from build123d import *

# Parameters (mm, degrees)
SKETCH1_W           = 45
SKETCH1_H           = 45
BOSS_EXTRUDE1_DEPTH = 48
SKETCH2_W           = 7
SKETCH2_H           = 3
CUT_EXTRUDE1_DEPTH  = 15
SKETCH3_R           = 3
CUT_EXTRUDE2_DEPTH  = 8
SKETCH4_W           = 18.249611446
SKETCH4_H           = 11.178416291
CUT_EXTRUDE3_DEPTH  = 2
BOSS_EXTRUDE2_DEPTH = 5


with BuildPart() as part:
    # Sketch1 → Boss-Extrude1 (new body)
    with BuildSketch(Plane(origin=(0, 0, 0), x_dir=(1, 0, 0), z_dir=(0, 1, 0))):
        with Locations((22.5, 22.5)):
            Rectangle(SKETCH1_W, SKETCH1_H)
    extrude(amount=BOSS_EXTRUDE1_DEPTH)

    # Sketch2 → Cut-Extrude1 (cut)
    with BuildSketch(Plane(origin=(0, 48, 0), x_dir=(1, 0, 0), z_dir=(0, 1, 0))):
        with Locations((5.5, 1.5)):
            Rectangle(SKETCH2_W, SKETCH2_H)
        with Locations((14, 1.5)):
            Rectangle(SKETCH2_W, SKETCH2_H)
        with Locations((22.5, 1.5)):
            Rectangle(SKETCH2_W, SKETCH2_H)
        with Locations((31, 1.5)):
            Rectangle(SKETCH2_W, SKETCH2_H)
        with Locations((39.5, 1.5)):
            Rectangle(SKETCH2_W, SKETCH2_H)
        with Locations((39.5, 43.5)):
            Rectangle(SKETCH2_W, SKETCH2_H)
        with Locations((31, 43.5)):
            Rectangle(SKETCH2_W, SKETCH2_H)
        with Locations((22.5, 43.5)):
            Rectangle(SKETCH2_W, SKETCH2_H)
        with Locations((14, 43.5)):
            Rectangle(SKETCH2_W, SKETCH2_H)
        with Locations((5.5, 43.5)):
            Rectangle(SKETCH2_W, SKETCH2_H)
    extrude(amount=-CUT_EXTRUDE1_DEPTH, mode=Mode.SUBTRACT)

    # Sketch3 → Cut-Extrude2 (cut)
    with BuildSketch(Plane(origin=(0, 48, 0), x_dir=(1, 0, 0), z_dir=(0, 1, 0))):
        with Locations((5.5, 8)):
            Circle(SKETCH3_R)
        with Locations((14, 8)):
            Circle(SKETCH3_R)
        with Locations((22.5, 8)):
            Circle(SKETCH3_R)
        with Locations((31, 8)):
            Circle(SKETCH3_R)
        with Locations((39.5, 8)):
            Circle(SKETCH3_R)
        with Locations((39.5, 37)):
            Circle(SKETCH3_R)
        with Locations((31, 37)):
            Circle(SKETCH3_R)
        with Locations((22.5, 37)):
            Circle(SKETCH3_R)
        with Locations((14, 37)):
            Circle(SKETCH3_R)
        with Locations((5.5, 37)):
            Circle(SKETCH3_R)
    extrude(amount=-CUT_EXTRUDE2_DEPTH, mode=Mode.SUBTRACT)

    # Sketch4 → Cut-Extrude3 (cut)
    with BuildSketch(Plane(origin=(0, 48, 0), x_dir=(1, 0, 0), z_dir=(0, 1, 0))):
        with Locations((21.737835253, 23.050452318)):
            Rectangle(SKETCH4_W, SKETCH4_H)
    extrude(amount=-CUT_EXTRUDE3_DEPTH, mode=Mode.SUBTRACT)

    # Sketch5 → Boss-Extrude2 (add)
    with BuildSketch(Plane(origin=(0, 0, 0), x_dir=(-1, 0, 0), z_dir=(0, -1, 0))):
        with BuildLine():
            Line((-42.5, 48), (-42.5, 51))
            Line((-42.5, 51), (-45, 51))
            Line((-45, 51), (-45, 45))
            Line((-45, 45), (-36, 45))
            Line((-36, 45), (-36, 51))
            Line((-36, 51), (-38.5, 51))
            Line((-38.5, 51), (-38.5, 48))
            ThreePointArc((-38.5, 48), (-40.5, 46), (-42.5, 48))
        make_face()
        with BuildLine():
            Line((-45, 0), (-36, 0))
            Line((-36, 0), (-36, -6))
            Line((-36, -6), (-38.5, -6))
            Line((-38.5, -6), (-38.5, -3))
            ThreePointArc((-38.5, -3), (-40.5, -1), (-42.5, -3))
            Line((-42.5, -3), (-42.5, -6))
            Line((-42.5, -6), (-45, -6))
            Line((-45, -6), (-45, 0))
        make_face()
    extrude(amount=-BOSS_EXTRUDE2_DEPTH)


solid = part.part
Input: part model. Units: mm. Frame: model coordinates. A direction names the side the tool comes from. Give positions to 0.01 mm unless a question says otherwise; leave off trailing zeros. Loops run counter-clockwise (first coordinate to the right, second up) from the corner with the lowest first, then second, coordinate; pieces in that order, holes last. Notation, with made-up numbers: M 34,51.25 L 86,51.25 A4 cw 86,58.25 Z; hole C -11.75,50.25 d9. An arc over 180 degrees is marked long. Use CSV: the item, a comma, the result in double quotes.
(1) Section C-C, the plane x = 5.5. Return loops of the section in (y, z).
Outcome:
outline,"M 0,-45 L 33,-45 L 33,-42 L 48,-42 L 48,-40 L 40,-40 L 40,-34 L 48,-34 L 48,-11 L 40,-11 L 40,-5 L 48,-5 L 48,-3 L 33,-3 L 33,0 L 0,0 Z"
(2) Pin query (flat end, axial travel): P1, Ø1.5, axis at y = 2, z = -50, coming from the -X side; P2, Ø5.5, axis at x = 39.5, z = -37, coming from the +Y side; P3, Ø7.5, axis at x = 24, y = 44, coming from the +Z side. Return the tip coordinate at first contact, or that it passes through.
Outcome:
P1,"stops at x = 36"
P2,"stops at y = 40"
P3,"stops at z = 0"
(3) Section B-B, the plane z = -8. Return loops of the section in (x, y).
Outcome:
outline,"M 0,0 L 45,0 L 45,48 L 42.5,48 L 42.5,40 L 36.5,40 L 36.5,48 L 34,48 L 34,40 L 28,40 L 28,48 L 25.5,48 L 25.5,40 L 19.5,40 L 19.5,48 L 17,48 L 17,40 L 11,40 L 11,48 L 8.5,48 L 8.5,40 L 2.5,40 L 2.5,48 L 0,48 Z"
(4) Pull-direction query (Z, two-part tool) for faces 1 (the face through (2, 41, -1)), 2 (the face through (31, 40, -8)), 3 (the face through (22, 41, -42)), 4 (the face through (28, 44, -8)); classes: pulls with the +Z half, pulls with the -Z half, needs draft (parallel to the pull), parting line crosses it, or undercut.
Outcome:
face 1,"needs draft"
face 2,"undercut"
face 3,"pulls with the -Z half"
face 4,"undercut"
(5) Section A-A, the plane x = 14. Return loops of the section in (y, z), plus the area to 3 significant figures.
Outcome:
outline,"M 0,-45 L 33,-45 L 33,-42 L 48,-42 L 48,-40 L 40,-40 L 40,-34 L 48,-34 L 48,-28.64 L 46,-28.64 L 46,-17.46 L 48,-17.46 L 48,-11 L 40,-11 L 40,-5 L 48,-5 L 48,-3 L 33,-3 L 33,0 L 0,0 Z"
area,"1,950 mm²"
(6) Section D-D, the plane y = 10.5. Return loops of the section in (x, z), plus the area to 4 significant figures.
Outcome:
outline,"M 0,-45 L 45,-45 L 45,0 L 0,0 Z"
area,"2,025 mm²"
(7) Set-up query: faces 5 (the face through (19.5, 44.1, -8.1)), 6 (the face through (10.5, 41, -43)), 7 (the face through (5, 33, -2)). Return all of +Z, -Z, +X, -X, +Y, -Y with unobstructed straight access to the full face (end or side cutting, diameter ignored); none if empty.
Outcome:
face 5,"+Y"
face 6,"-Z, +Y"
face 7,"+Z, +Y"
(8) Material intervals for L1, parallel to X at y = 42, z = -8; L2, parallel to Z at x = 22.5, y = 43.5; L3, parallel to X at y = 46, z = -44, sorted ascending. Write a range as [from, to].
Outcome:
L1,"x = [0, 2.5], [8.5, 11], [17, 19.5], [25.5, 28], [34, 36.5], [42.5, 45]"
L2,"z = [-42, -40], [-34, -11], [-5, -3]"
L3,"x = [0, 2], [9, 10.5], [17.5, 19], [26, 27.5], [34.5, 36], [43, 45]"
